Can you work these out from the drawing? Everything is in mm from the part's minimum corner. A direction names the side the tool comes from. Coordinates: 2 decimals unless noted, no trailing zeros. Order: outer loops, then holes, each group sorted by start corner. A loop starts at its lowest first (then second) coordinate and runs counter-clockwise, first axis right, second up. Notation, with made-up numbers: (87, 73) - (141, 73) arc R22 ccw to (141, 98) - close; hole circle Ø4 at (36, -28). An arc over 180 degrees is marked (long way). Use CSV: the item, a comma, the result in double quotes. Start each with the question number.
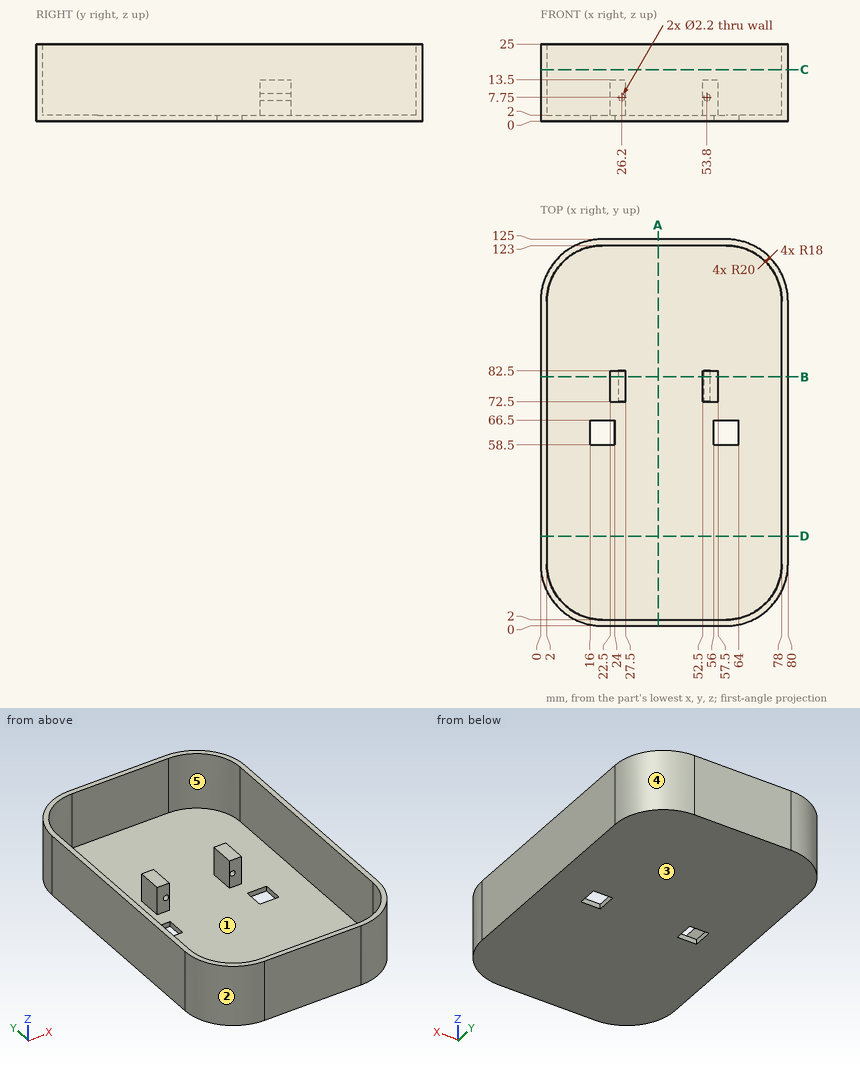
Item 1: We'd pull the mould along Y, two halves only. Please class the marked faces 1, 2 and 3: released by +Y, released by -Y, zero draft, split by the parting line, or undercut.
Item 2: For the marked faces 4 and 5, which set-ups out of +Z, -Z, +X, -X, +Y, -Y let a thin tool reach every point of the face, with its end or its side?
Item 3: Suppose I cut it at D-D on y = 29. Write out the boundary of the cut face in (x, z).
Item 4: Please list where these lines run through material, in increasing order: line 1 along Z through (x, y) = (26.2, 76.75); line 2 along Y through (x, z) = (40, 17.5); line 3 along X through (y, z) = (40, 6.5). Write a range as from..to.
Item 5: Suppose I cut it at C-C on z = 16.75. Write out the boundary of the cut face in (x, y).
Item 6: For pin 1 Ø1.5 at (x, y) = (55, 51) entering from +Z; pin 2 Ø0.6 at (x, z) = (61.5, 1) entering from -Y, each with a flat end and sliding along its axis, tell me the tip position at first contact or that it passes through.
Item 7: Suppose I cut it at B-B on y = 80.5. Write out the boundary of the cut face in (x, z), then the cut area to 3 significant figures.
Item 8: Suppose I cut it at A-A on x = 38. Write out the boundary of the cut face in (y, z).
Here are the results:
1,face 1,"undercut"
1,face 2,"released by -Y"
1,face 3,"zero draft"
2,face 4,"+Z, -Z, +X, +Y"
2,face 5,"+Z"
3,outline,"(0, 0) - (80, 0) - (80, 25) - (78, 25) - (78, 2) - (2, 2) - (2, 25) - (0, 25) - close"
4,line 1,"0..6.65, 8.85..13.5"
4,line 2,"0..2, 123..125"
4,line 3,"0..2, 78..80"
5,outline,"(0, 20) arc R20 ccw to (20, 0) - (60, 0) arc R20 ccw to (80, 20) - (80, 105) arc R20 ccw to (60, 125) - (20, 125) arc R20 ccw to (0, 105) - close; hole (2, 20) arc R18 ccw to (20, 2) - (60, 2) arc R18 ccw to (78, 20) - (78, 105) arc R18 ccw to (60, 123) - (20, 123) arc R18 ccw to (2, 105) - close"
6,pin 1,"z = 2"
6,pin 2,"y = 0.04"
7,outline,"(0, 0) - (80, 0) - (80, 25) - (78, 25) - (78, 2) - (57.5, 2) - (57.5, 13.5) - (52.5, 13.5) - (52.5, 2) - (27.5, 2) - (27.5, 13.5) - (22.5, 13.5) - (22.5, 2) - (2, 2) - (2, 25) - (0, 25) - close; hole circle Ø2.2 at (26.2, 7.75); hole circle Ø2.2 at (53.8, 7.75)"
7,area,"359 mm^2"
8,outline,"(0, 0) - (125, 0) - (125, 25) - (123, 25) - (123, 2) - (2, 2) - (2, 25) - (0, 25) - close"
